Geometry check sheet. Reference: the model listing, model coordinates, mm. A direction names the side the tool comes from. Give positions to 0.01 mm unless a question says otherwise; leave off trailing zeros. Write each loop counter-clockwise with the first axis right and the second up, starting at its lowest first coordinate (ties: lowest second). Pieces come first, ordered by that corner, then holes. Notation, with made-up numbers: (-5, 30) -> (2, 30) arc R18 cw to (2, 48) -> close; hole circle Ø9 at (47.25, 27). An arc over 180 degrees is marked (long way). One line per item, written item: value.
from build123d import *

# Parameters (mm, degrees)
F0_W      = 10
F0_H      = 3.5
F1_DEPTH  = 20
F2_R      = 3
F3_DEPTH  = 3.501
F6_R      = 5
F9_DEPTH  = 18
F10_DEPTH = 20.001
F11_R     = 5


with BuildPart() as f1:
    # F0 (on Front) → F1 (new body)
    with BuildSketch(Plane.XZ):
        with Locations((-70, 1.75)):
            Rectangle(F0_W, F0_H)
        Polygon((-65, 0), (0, 0), (0, 3.5), (0, 32), (-65, 32), (-65, 3.5), align=None)
        with Locations((5, 1.75)):
            Rectangle(F0_W, F0_H)
    extrude(amount=F1_DEPTH)

    # F2 (on face) → F3 (cut, through all)
    with BuildSketch(Plane.XY.offset(3.5)):
        with Locations((5, -10)):
            Circle(F2_R)
    f3 = extrude(amount=-F3_DEPTH, mode=Mode.SUBTRACT)

    # F5: F3 across plane
    add(f3.mirror(Plane.YZ.offset(-32.5)), mode=Mode.SUBTRACT)

    # F6
    f6_edges = [f1.edges().sort_by_distance(p)[0] for p in [
        (0, -10, 32),
        (-65, -10, 32),
    ]]
    fillet(f6_edges, radius=F6_R)

    # F8 (on face) → F9 (cut)
    with BuildSketch(Plane.XZ.offset(20)):
        with BuildLine():
            Line((-58.5, 2.5), (-6.5, 2.5))
            ThreePointArc((-6.5, 2.5), (-5.0857864376, 3.0857864376), (-4.5, 4.5))
            Line((-4.5, 4.5), (-4.5, 27.5))
            ThreePointArc((-4.5, 27.5), (-5.0857864376, 28.9142135624), (-6.5, 29.5))
            Line((-6.5, 29.5), (-58.5, 29.5))
            ThreePointArc((-58.5, 29.5), (-59.9142135624, 28.9142135624), (-60.5, 27.5))
            Line((-60.5, 27.5), (-60.5, 4.5))
            ThreePointArc((-60.5, 4.5), (-59.9142135624, 3.0857864376), (-58.5, 2.5))
        make_face()
    extrude(amount=-F9_DEPTH, mode=Mode.SUBTRACT)

    # F7 (on face) → F10 (cut, through all)
    with BuildSketch(Plane(origin=(0, 0, 0), x_dir=(-1, 0, 0), z_dir=(0, 1, 0))):
        with BuildLine():
            ThreePointArc((15.5251769957, 13.4682242014), (16.9896430898, 9.9326902954), (20.5251769957, 8.4682242014))
            Line((20.5251769957, 8.4682242014), (44.4748230043, 8.4682242014))
            ThreePointArc((44.4748230043, 8.4682242014), (48.0103569102, 9.9326902954), (49.4748230043, 13.4682242014))
            Line((49.4748230043, 13.4682242014), (49.4748230043, 18.5317757986))
            ThreePointArc((49.4748230043, 18.5317757986), (48.0103569102, 22.0673097046), (44.4748230043, 23.5317757986))
            Line((44.4748230043, 23.5317757986), (20.5251769957, 23.5317757986))
            ThreePointArc((20.5251769957, 23.5317757986), (16.9896430898, 22.0673097046), (15.5251769957, 18.5317757986))
            Line((15.5251769957, 18.5317757986), (15.5251769957, 13.4682242014))
        make_face()
    extrude(amount=-F10_DEPTH, mode=Mode.SUBTRACT)

    # F11
    f11_edges = [f1.edges().sort_by_distance(p)[0] for p in [
        (-75, -20, 1.75),
        (-75, 0, 1.75),
        (10, -20, 1.75),
        (10, 0, 1.75),
    ]]
    fillet(f11_edges, radius=F11_R)


solid = f1.part
1) Mould release check, pull along Z, two halves, no side actions. Record for faces 1 (the flat face through (-33, -10, 0)), 2 (the cylindrical face through (-17.03, -0.99, 22.11)), 3 (the cylindrical face through (8, -1, 2)), 4 (the cylindrical face through (-1, -10, 30)): released by +Z, released by -Z, zero draft, split by the parting line, or undercut.
Verdict:
face 1: released by -Z
face 2: undercut
face 3: zero draft
face 4: released by +Z
2) Sectioned sample at B-B on x = -30.5. Record the cut outline in (y, z), plus the area to 3 significant figures.
Verdict:
outline: (-20, 0) -> (0, 0) -> (0, 8.47) -> (-2, 8.47) -> (-2, 2.5) -> (-20, 2.5) -> close; (-20, 29.5) -> (-2, 29.5) -> (-2, 23.53) -> (0, 23.53) -> (0, 32) -> (-20, 32) -> close
area: 124 mm^2
3) Tool access check on faces 5 (the cylindrical face through (-47.97, -0.99, 9.89)), 6 (the flat face through (0, -10, 15)), 7 (the flat face through (-35, -20, 2)), 8 (the cylindrical face through (-5.07, -11.13, 28.9)). Record the directions out of +Z, -Z, +X, -X, +Y, -Y that give a thin tool (end or side, any length) a straight path to the whole face; none if there is none.
Verdict:
face 5: +Y, -Y
face 6: +Z, +X, +Y, -Y
face 7: +Z, -Z, +X, -X, -Y
face 8: -Y
4) Depth check by flat-ended pin: pin 1 Ø5.5 at (y, z) = (-11.5, 19) entering from -X; pin 2 Ø3 at (x, y) = (-71, -12.5) entering from +Z; pin 3 Ø0.6 at (x, y) = (-29.5, -1.5) entering from -Z; pin 4 Ø3 at (x, z) = (-36, 9) entering from -Y. Enter the tip coordinate at first touch or a pass-through.
Verdict:
pin 1: x = -65
pin 2: z = 3.5
pin 3: z = 0
pin 4: y = -2
5) Sectioned sample at A-A on y = -10. Record the cut outline in (x, z).
Verdict:
outline: (-75, 0) -> (-73, 0) -> (-73, 3.5) -> (-75, 3.5) -> close; (-67, 0) -> (2, 0) -> (2, 3.5) -> (0, 3.5) -> (0, 27) arc R5 ccw to (-5, 32) -> (-60, 32) arc R5 ccw to (-65, 27) -> (-65, 3.5) -> (-67, 3.5) -> close; (8, 0) -> (10, 0) -> (10, 3.5) -> (8, 3.5) -> close; hole (-60.5, 4.5) arc R2 ccw to (-58.5, 2.5) -> (-6.5, 2.5) arc R2 ccw to (-4.5, 4.5) -> (-4.5, 27.5) arc R2 ccw to (-6.5, 29.5) -> (-58.5, 29.5) arc R2 ccw to (-60.5, 27.5) -> close
6) Sectioned sample at C-C on z = 20.5. Record the cut outline in (x, y).
Verdict:
outline: (-65, -20) -> (-60.5, -20) -> (-60.5, -2) -> (-49.07, -2) -> (-49.07, 0) -> (-65, 0) -> close; (-15.93, -2) -> (-4.5, -2) -> (-4.5, -20) -> (0, -20) -> (0, 0) -> (-15.93, 0) -> close
7) Scan lines: probe 1 along X at (y, z) = (-14.75, 9); probe 2 along Z at (x, y) = (-13.5, -9); probe 3 along X at (y, z) = (-1.75, 14.5). Record each from-to range of solid material in increasing order.
Verdict:
probe 1: -65 to -60.5, -4.5 to 0
probe 2: 0 to 2.5, 29.5 to 32
probe 3: -65 to -49.47, -15.53 to 0
8) Sectioned sample at D-D on x = -9.5. Record the cut outline in (y, z).
Verdict:
outline: (-20, 0) -> (0, 0) -> (0, 32) -> (-20, 32) -> (-20, 29.5) -> (-2, 29.5) -> (-2, 2.5) -> (-20, 2.5) -> close
